from build123d import *

# Parameters (mm, degrees)
F0_R     = 1.0922
F0_R_2   = 1.5875
F1_DEPTH = 6.35


with BuildPart() as f1:
    # F0 (on Front) → F1 (new body)
    with BuildSketch(Plane.XZ):
        with BuildLine():
            Line((66.675, 31.75), (-66.675, 31.75))
            ThreePointArc((-66.675, 31.75), (-67.604936, 29.504936), (-69.85, 28.575))
            Line((-69.85, 28.575), (-69.85, 0))
            Line((-69.85, 0), (-60.325, 0))
            Line((-60.325, 0), (-60.325, 20.32))
            Line((-60.325, 20.32), (-9.525, 20.32))
            Line((-9.525, 20.32), (-9.525, 25.4))
            Line((-9.525, 25.4), (9.525, 25.4))
            Line((9.525, 25.4), (9.525, 20.32))
            Line((9.525, 20.32), (60.325, 20.32))
            Line((60.325, 20.32), (60.325, 0))
            Line((60.325, 0), (69.85, 0))
            Line((69.85, 0), (69.85, 28.575))
            ThreePointArc((69.85, 28.575), (67.604936, 29.504936), (66.675, 31.75))
        make_face()
        with Locations((-56.261, 22.86)):
            Circle(F0_R, mode=Mode.SUBTRACT)
        with Locations((-57.404, 27.178)):
            Circle(F0_R_2, mode=Mode.SUBTRACT)
        with Locations((56.261, 22.86)):
            Circle(F0_R, mode=Mode.SUBTRACT)
        with Locations((57.404, 27.178)):
            Circle(F0_R_2, mode=Mode.SUBTRACT)
        with BuildLine():
            Line((-60.325, 0), (-69.85, 0))
            Line((-69.85, 0), (-69.85, -28.575))
            ThreePointArc((-69.85, -28.575), (-67.604936, -29.504936), (-66.675, -31.75))
            Line((-66.675, -31.75), (66.675, -31.75))
            ThreePointArc((66.675, -31.75), (67.604936, -29.504936), (69.85, -28.575))
            Line((69.85, -28.575), (69.85, 0))
            Line((69.85, 0), (60.325, 0))
            Line((60.325, 0), (60.325, -20.32))
            Line((60.325, -20.32), (-60.325, -20.32))
            Line((-60.325, -20.32), (-60.325, 0))
        make_face()
        with Locations((-57.404, -27.178)):
            Circle(F0_R_2, mode=Mode.SUBTRACT)
        with Locations((-56.261, -22.86)):
            Circle(F0_R, mode=Mode.SUBTRACT)
        with Locations((57.404, -27.178)):
            Circle(F0_R_2, mode=Mode.SUBTRACT)
        with Locations((56.261, -22.86)):
            Circle(F0_R, mode=Mode.SUBTRACT)
    extrude(amount=F1_DEPTH)


solid = f1.part
Work out the finished part from the listing and answer in its coordinate system (mm). A direction names the side the tool comes from. Give positions to 0.01 mm unless a question says otherwise; leave off trailing zeros. Write each loop counter-clockwise with the first axis right and the second up, starting at its lowest first coordinate (ties: lowest second). Pieces come first, ordered by that corner, then holes.
Q1. Given pin 1 (6 mm diameter, centred on x = 42.5, z = -16.5, fed in from +Y), flat-ended and moving along its own axis, determine where the tip first touches the part or whether it passes through.
Answer:
pin 1: passes through
Q2. The part is cut by section C-C on y = -3. State how many separate pieces and enclosed holes the cut face has, and give its area (3 significant figures).
Answer:
separate pieces: 1
enclosed holes: 9
area: 3,790 mm2
Q3. A tool of negligible diameter and unlimited length cuts with its end or side. For faces 5 (the face through (-60.325, -3, 0)), 6 (the face through (-69.85, -3, 0)), from which of +Z, -Z, +X, -X, +Y, -Y can it reach the whole face along a straight path? Write none if from no direction.
Answer:
face 5: +Y, -Y
face 6: +Z, -Z, -X, +Y, -Y
Q4. The part is cut by section A-A on z = -18.5. Give the vertices of the cut face in (x, y) (3 decimals), and give its area (3 significant figures).
Answer:
outline: (-69.85, -6.35) - (-60.325, -6.35) - (-60.325, 0) - (-69.85, 0) - close; (60.325, -6.35) - (69.85, -6.35) - (69.85, 0) - (60.325, 0) - close
area: 121 mm2
Q5. Straight lines are drawn through the part: L1, parallel to X at y = -0.5, z = -14.5 (3 decimals); L2, parallel to Z at x = 12.5, y = -2; L3, parallel to Z at x = -0.5, y = -3.75. For each, find the intervals that lie inside material, in ascending order.
Answer:
L1: x = -69.85 to -60.325, 60.325 to 69.85
L2: z = -31.75 to -20.32, 20.32 to 31.75
L3: z = -31.75 to -20.32, 25.4 to 31.75
Q6. The part is cut by section B-B on x = 41. Give the vertices of the cut face in (y, z), and give its area (3 significant figures).
Answer:
outline: (-6.35, -31.75) - (0, -31.75) - (0, -20.32) - (-6.35, -20.32) - close; (-6.35, 20.32) - (0, 20.32) - (0, 31.75) - (-6.35, 31.75) - close
area: 145 mm2
Q7. For a pull along X with two mould halves and no side action, classify faces 1 (the face through (69.85, -3, 0)), 2 (the face through (-67.58, -3.13, 29.53)), 3 (the face through (-55.89, -3.13, -26.7)), 4 (the face through (0, -3, 25.4)) as released by +X, released by -X, zero draft, split by the parting line, or undercut.
Answer:
face 1: released by +X
face 2: released by -X
face 3: undercut
face 4: undercut
